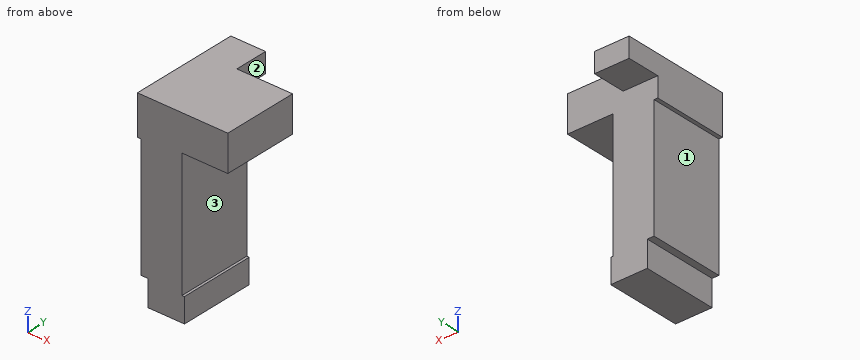
from build123d import *

# Parameters (mm, degrees)
BOSS_EXTRUDE1_DEPTH = 610
SKETCH2_W           = 280
SKETCH2_H           = 160
BOSS_EXTRUDE2_DEPTH = 270


with BuildPart() as part:
    # Sketch1 → Boss-Extrude1 (new body)
    with BuildSketch(Plane(origin=(0, 0, 0), x_dir=(1, 0, 0), z_dir=(0, 1, 0))):
        Polygon((730, 290), (360, 290), (360, 1312.957638722), (380, 1312.957638722), (380, 1510), (85, 1510), (85, 1300), (30, 1300), (30, 320), (0, 320), (0, 0), (730, 0), align=None)
    extrude(amount=BOSS_EXTRUDE1_DEPTH)

    # Sketch2 → Boss-Extrude2 (add)
    with BuildSketch(Plane(origin=(0, 610, 0), x_dir=(1, 0, 0), z_dir=(0, 1, 0))):
        with Locations((140, 80)):
            Rectangle(SKETCH2_W, SKETCH2_H)
    extrude(amount=BOSS_EXTRUDE2_DEPTH)


solid = part.part
Could you check a few things on this model? Use its own coordinates, in mm. Face numbers are marked on the shaded views. A direction names the side the tool comes from. Give positions to 0.01 mm unless a question says otherwise; leave off trailing zeros. Order: outer loops, then holes, each group sorted by start corner. A loop starts at its lowest first (then second) coordinate and runs counter-clockwise, first axis right, second up.
Item 1: If we section it at B-B, the plane y = 585: Write out the boundary of the cut face in (x, z).
Item 2: If we section it at C-C, the plane x = 257: Write out the boundary of the cut face in (y, z), plus the area to 3 significant figures.
Item 3: I need wall thicknesses on line 1 (Z direction, x = 454, y = 292); line 2 (X direction, y = 364.5, z = -612); line 3 (X direction, y = 133.5, z = -1428). Which ranges of each line are inside material? Lowest first, please.
Item 4: If we section it at A-A, the plane z = -108: Write out the boundary of the cut face in (x, y), plus the area to 3 significant figures.
Item 5: For the marked faces 1, 2 and 3, which set-ups out of +Z, -Z, +X, -X, +Y, -Y let a thin tool reach every point of the face, with its end or its side?
Item 6: I'm going to push flat-ended pins straight in: pin 1 (10 mm diameter, centred on x = 488, y = 462, fed in from +Z); pin 2 (2 mm diameter, centred on y = 601.5, z = -445, fed in from -X); pin 3 (9 mm diameter, centred on x = 13.5, y = 226, fed in from -Z); pin 4 (12 mm diameter, centred on x = 208, z = -544, fed in from +Y). Where does each tip first touch, or does it pass through?
Item 7: If we section it at D-D, the plane y = 812: Write out the boundary of the cut face in (x, z), plus the area to 3 significant figures.
Values:
1. outline: (0, -320) - (30, -320) - (30, -1300) - (85, -1300) - (85, -1510) - (380, -1510) - (380, -1312.96) - (360, -1312.96) - (360, -290) - (730, -290) - (730, 0) - (0, 0) - close
2. outline: (0, -1510) - (610, -1510) - (610, -160) - (880, -160) - (880, 0) - (0, 0) - close
2. area: 964,000 mm2
3. line 1: z = -290 to 0
3. line 2: x = 30 to 360
3. line 3: x = 85 to 380
4. outline: (0, 0) - (730, 0) - (730, 610) - (280, 610) - (280, 880) - (0, 880) - close
4. area: 521,000 mm2
5. face 1: -Z, -X, +Y, -Y
5. face 2: +Z, -Z, +X, +Y
5. face 3: +X, +Y, -Y
6. pin 1: stops at z = 0
6. pin 2: stops at x = 30
6. pin 3: stops at z = -320
6. pin 4: stops at y = 610
7. outline: (0, -160) - (280, -160) - (280, 0) - (0, 0) - close
7. area: 44,800 mm2
